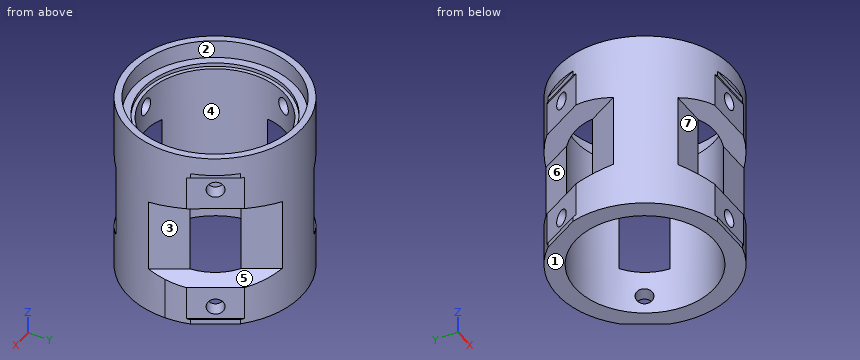
```python
from build123d import *

# Parameters (mm, degrees)
F0_R           = 24
F0_R_2         = 19
F1_DEPTH       = 50
F2_R           = 22.15
F3_DEPTH       = 5
F4_R           = 20
F5_DEPTH       = 1
F6_R           = 57.967167
F7_DEPTH       = 45
F9_DEPTH       = 25
F10_COUNT      = 3
F10_ANGLE      = 240
F12_R          = 2.25
F13_DEPTH      = 10
F13_DEPTH_BACK = 10
F14_COUNT      = 3
F14_ANGLE      = 240


with BuildPart() as f1:
    # F0 (on Top) → F1 (new body)
    with BuildSketch(Plane.XY):
        Circle(F0_R)
        Circle(F0_R_2, mode=Mode.SUBTRACT)
    extrude(amount=F1_DEPTH)

    # F2 (on face) → F3 (cut)
    with BuildSketch(Plane.XY.offset(50)):
        Circle(F2_R)
    extrude(amount=-F3_DEPTH, mode=Mode.SUBTRACT)

    # F4 (on face) → F5 (cut)
    with BuildSketch(Plane.XY.offset(45)):
        Circle(F4_R)
    extrude(amount=-F5_DEPTH, mode=Mode.SUBTRACT)

    # F6 (on Top) → F7 (cut)
    with BuildSketch(Plane.XY):
        Circle(F6_R)
        Polygon((0, 46.5), (40.270181, -23.25), (-40.270181, -23.25), align=None, mode=Mode.SUBTRACT)
    extrude(amount=F7_DEPTH, mode=Mode.SUBTRACT)


with BuildPart() as f9:
    # F8 (on Right) → F9 (new body, symmetric)
    with BuildSketch(Plane.YZ):
        Polygon((-23, 34.319851), (-23, 43.612687), (-27.333883, 45.190091), (-27.333883, -0.190091), (-23, 1.387313), (-23, 10.680149), (-18, 12.5), (-18, 22.5), (-18, 32.5), align=None)
    extrude(amount=F9_DEPTH, both=True)


with BuildPart() as f10_1:
    # F10: instance of F9
    add(f9.part.rotate(Axis((0, 0, 0), (0, 0, -1)), 1 * F10_ANGLE / (F10_COUNT - 1)))


with BuildPart() as f10_2:
    # F10: instance of F9
    add(f9.part.rotate(Axis((0, 0, 0), (0, 0, -1)), 2 * F10_ANGLE / (F10_COUNT - 1)))


with BuildPart() as f1_1:
    add(f1.part)

    # F11: cut F10_2, F10_1, F9
    add(f10_2.part, mode=Mode.SUBTRACT)
    add(f10_1.part, mode=Mode.SUBTRACT)
    add(f9.part, mode=Mode.SUBTRACT)


with BuildPart() as f13:
    # F12 (on face) → F13 (new body, two sides)
    with BuildSketch(Plane.XZ.offset(23)) as f13_sk:
        with Locations((0, 40)):
            Circle(F12_R)
        with Locations((0, 5)):
            Circle(F12_R)
    extrude(amount=-F13_DEPTH)
    extrude(f13_sk.sketch, amount=-F13_DEPTH_BACK)


with BuildPart() as f14_1:
    # F14: instance of F13
    add(f13.part.rotate(Axis((0, 0, 0), (0, 0, -1)), 1 * F14_ANGLE / (F14_COUNT - 1)))


with BuildPart() as f14_2:
    # F14: instance of F13
    add(f13.part.rotate(Axis((0, 0, 0), (0, 0, -1)), 2 * F14_ANGLE / (F14_COUNT - 1)))


with BuildPart() as f1_2:
    add(f1_1.part)

    # F15: cut F14_2, F14_1, F13
    add(f14_2.part, mode=Mode.SUBTRACT)
    add(f14_1.part, mode=Mode.SUBTRACT)
    add(f13.part, mode=Mode.SUBTRACT)


solid = f1_2.part
```
Verification items for the finished model (mm, model axes). Face numbers are marked on the shaded views. A direction names the side the tool comes from. Coordinates: 2 decimals unless noted, no trailing zeros. Write each loop counter-clockwise with the first axis right and the second up, starting at its lowest first coordinate (ties: lowest second). Pieces come first, ordered by that corner, then holes. Notation, with made-up numbers: M 46.25,20 L 91.25,20 A14 cw 91.25,41 Z; hole C 14.5,-35 d9. An arc over 180 degrees is marked long. Answer as a JSON object with one key per item and string values. Group by question number.
(1) Cross-section at C-C, the plane x = -5. Record the cut outline in (y, z), and give its area (3 significant figures).
(2) Material ranges on line 1 (Y direction, x = 0, z = 46); line 2 (Z direction, x = 0, y = -21.4); line 3 (Z direction, x = 0, y = -21.75), recorded low to high.
(3) Cross-section at A-A, the plane z = 16. Record the cut outline in (x, y).
(4) Gauge pin test, flat ends, axial feed: pin 1 (3 mm diameter, centred on y = 8, z = 7, fed in from -X); pin 2 (4 mm diameter, centred on x = 0, z = 40, fed in from +Y); pin 3 (10 mm diameter, centred on x = -2, z = 6, fed in from -Y); pin 4 (2 mm diameter, centred on x = 10, y = 14.5, fed in from -Z). Record the tip position at first contact, or that the pin passes through.
(5) Cross-section at B-B, the plane y = -8.5. Record the cut outline in (x, z).
(6) Release check for a two-part mould opening along X. For the marked faces 1, 2, 3 and 4 record: +X half, -X half, draft (parallel to the pull), parting line (faces both ways), or undercut.
(7) Tool access check on the marked faces 5, 6 and 7. Record the directions out of +Z, -Z, +X, -X, +Y, -Y that give a thin tool (end or side, any length) a straight path to the whole face; none if there is none.
(8) Cross-section at D-D, the plane x = 0. State how many separate pieces and enclosed holes the cut face has, and give its area (3 significant figures).
Reply:
{
 "1": {"outline": "M -23.47,45 L -23.25,45 L -23.25,43.7 L -23,43.61 L -23,34.32 L -18.33,32.62 L -18.33,44 L -19.36,44 L -19.36,45 L -21.58,45 L -21.58,50 L -23.47,50 Z; M -23.25,0 L -18.33,0 L -18.33,12.38 L -23,10.68 L -23,1.39 L -23.25,1.3 Z; M 18.33,0 L 23.47,0 L 23.47,50 L 21.58,50 L 21.58,45 L 19.36,45 L 19.36,44 L 18.33,44 Z", "area": "357 mm²"},
 "2": {"line 1": "-24 to -22.15, 22.15 to 24", "line 2": "0 to 2.75, 7.25 to 11.26, 33.74 to 37.75, 42.25 to 45", "line 3": "0 to 2.75, 7.25 to 11.14, 33.86 to 37.75, 42.25 to 45"},
 "3": {"outline": "M -23.53,-4.75 A24 ccw -15.87,-18 L -6.08,-18 A19 cw -18.63,3.73 Z; M -12.55,14.27 A19 cw 12.55,14.27 L 7.65,22.75 A24 ccw -7.65,22.75 Z; M 6.08,-18 L 15.87,-18 A24 ccw 23.53,-4.75 L 18.63,3.73 A19 cw Z"},
 "4": {"pin 1": "x = -22.81", "pin 2": "y = 24", "pin 3": "y = -23.25", "pin 4": "through"},
 "5": {"outline": "M -22.44,0 L -16.99,0 L -16.99,44 L -18.1,44 L -18.1,45 L -20.45,45 L -20.45,50 L -22.44,50 Z; M 16.99,0 L 22.44,0 L 22.44,50 L 20.45,50 L 20.45,45 L 18.1,45 L 18.1,44 L 16.99,44 Z"},
 "6": {"face 1": "draft", "face 2": "undercut", "face 3": "+X half", "face 4": "undercut"},
 "7": {"face 5": "+X, +Y", "face 6": "-X, +Y", "face 7": "+X, -X, -Y"},
 "8": {"separate pieces": "5", "enclosed holes": "0", "area": "297 mm²"}
}
